```python
from build123d import *

# Parameters (mm, degrees)
SKETCH1_W           = 158.5
SKETCH1_H           = 104
SKETCH1_W_2         = 62.25
SKETCH1_H_2         = 68
BOSS_EXTRUDE1_DEPTH = 1.2
SKETCH2_W           = 4
SKETCH2_H           = 10
BOSS_EXTRUDE2_DEPTH = 2
FILLET1_R           = 2
SKETCH3_W           = 10
SKETCH3_H           = 9
BOSS_EXTRUDE3_DEPTH = 5
SKETCH4_R           = 1.3
CUT_EXTRUDE1_DEPTH  = 5
CUT_EXTRUDE2_DEPTH  = 3.8
FILLET2_R           = 5
FILLET3_R           = 2
SKETCH6_W           = 98
SKETCH6_H           = 10
BOSS_EXTRUDE4_DEPTH = 0.8
SKETCH8_W           = 16
SKETCH8_H           = 6
BOSS_EXTRUDE5_DEPTH = 2
SKETCH9_W           = 6
SKETCH9_H           = 10
SKETCH9_W_2         = 3
SKETCH9_H_2         = 9.8
BOSS_EXTRUDE6_DEPTH = 2.8
FILLET4_R           = 3
SKETCH11_W          = 10
SKETCH11_H          = 71
BOSS_EXTRUDE7_DEPTH = 2
BOSS_EXTRUDE8_DEPTH = 1.2


# Some blends are built 0.0001 mm under size
with BuildPart() as part:
    # Sketch1 → Boss-Extrude1 (new body)
    with BuildSketch(Plane(origin=(0, 0, 0), x_dir=(1, 0, 0), z_dir=(0, 1, 0))):
        with Locations((79.25, 52)):
            Rectangle(SKETCH1_W, SKETCH1_H)
        with Locations((119.375, 54)):
            Rectangle(SKETCH1_W_2, SKETCH1_H_2, mode=Mode.SUBTRACT)
        with Locations((47.125, 54)):
            Rectangle(SKETCH1_W_2, SKETCH1_H_2, mode=Mode.SUBTRACT)
    extrude(amount=BOSS_EXTRUDE1_DEPTH)

    # Sketch2 → Boss-Extrude2 (add)
    with BuildSketch(Plane.XZ):
        with Locations((149.5, -104)):
            Rectangle(SKETCH2_W, SKETCH2_H)
        with Locations((48, -104)):
            Rectangle(SKETCH2_W, SKETCH2_H)
    extrude(amount=BOSS_EXTRUDE2_DEPTH)

    # Fillet1
    fillet1_edges = [part.edges().sort_by_distance(p)[0] for p in [
        (50, 0, -101.5),
        (46, 0, -101.5),
        (147.5, 0, -101.5),
        (151.5, 0, -101.5),
    ]]
    fillet(fillet1_edges, radius=FILLET1_R - 0.0001)  # a hair under: the kernel refuses the full size

    # Sketch3 → Boss-Extrude3 (add)
    with BuildSketch(Plane(origin=(0, 0, -104), x_dir=(-1, 0, 0), z_dir=(0, 0, -1))):
        with Locations((-95.75, -3.3)):
            Rectangle(SKETCH3_W, SKETCH3_H)
    extrude(amount=-BOSS_EXTRUDE3_DEPTH)

    # Sketch4 → Cut-Extrude1 (cut)
    with BuildSketch(Plane(origin=(0, 0, -104), x_dir=(-1, 0, 0), z_dir=(0, 0, -1))):
        with Locations((-95.75, -3.3)):
            Circle(SKETCH4_R)
    extrude(amount=-CUT_EXTRUDE1_DEPTH, mode=Mode.SUBTRACT)

    # Sketch5 → Cut-Extrude2 (cut)
    with BuildSketch(Plane.XY.offset(-99)):
        with BuildLine():
            Line((92.25, -3.3), (92.25, -7.8))
            Line((92.25, -7.8), (99.25, -7.8))
            Line((99.25, -7.8), (99.25, -3.3))
            ThreePointArc((99.25, -3.3), (95.75, 0.2), (92.25, -3.3))
        make_face()
    extrude(amount=-CUT_EXTRUDE2_DEPTH, mode=Mode.SUBTRACT)

    # Fillet2
    fillet2_edges = [part.edges().sort_by_distance(p)[0] for p in [
        (100.75, 0, -101.5),
        (90.75, 0, -101.5),
    ]]
    fillet(fillet2_edges, radius=FILLET2_R)

    # Fillet3
    fillet3_edges = [part.edges().sort_by_distance(p)[0] for p in [
        (90.75, -7.8, -101.5),
        (100.75, -7.8, -101.5),
    ]]
    fillet(fillet3_edges, radius=FILLET3_R)

    # Sketch6 → Boss-Extrude4 (add)
    with BuildSketch(Plane.XZ):
        with Locations((109.5, -10.2)):
            Rectangle(SKETCH6_W, SKETCH6_H)
    extrude(amount=BOSS_EXTRUDE4_DEPTH)

    # Sketch8 → Boss-Extrude5 (add)
    with BuildSketch(Plane.XZ):
        with Locations((160.5, -10.2)):
            Rectangle(SKETCH8_W, SKETCH8_H)
    extrude(amount=BOSS_EXTRUDE5_DEPTH)

    # Sketch9 → Boss-Extrude6 (add)
    with BuildSketch(Plane.XZ):
        with Locations((155.5, -10.2)):
            Rectangle(SKETCH9_W, SKETCH9_H)
        with Locations((59, -10.1)):
            Rectangle(SKETCH9_W_2, SKETCH9_H_2)
    extrude(amount=BOSS_EXTRUDE6_DEPTH)

    # Fillet4
    # the kernel refuses this fillet: 3 mm, written as the material it adds along each edge
    with BuildSketch(Plane(origin=(57.5, 0, -5.2), x_dir=(-1, 0, 0), z_dir=(0, 0, -1))) as fillet4_piece_1:
        with BuildLine():
            CenterArc((2.993325909, -3), FILLET4_R, 90, 86.177446271)
            Line((0, -2.8), (-0.059866518, -2.796))
            ThreePointArc((-0.059866518, -2.796), (-0.06, -1.4), (-0.06, 0))
            Line((-0.06, 0), (0, 0.06))
            Line((0, 0.06), (2.993325909, 0.06))
            Line((2.993325909, 0.06), (2.993325909, 0))
        make_face()
    extrude(amount=9.8)

    # Sketch11 → Boss-Extrude7 (add)
    with BuildSketch(Plane.XZ):
        with Locations((9, -35.5)):
            Rectangle(SKETCH11_W, SKETCH11_H)
    extrude(amount=BOSS_EXTRUDE7_DEPTH)

    # Sketch12 → Boss-Extrude8 (add)
    with BuildSketch(Plane(origin=(0, 1.2, 0), x_dir=(1, 0, 0), z_dir=(0, 1, 0))):
        with BuildLine():
            Line((22.585033293, 82.977390915), (39.739539441, 64.185732728))
            ThreePointArc((39.739539441, 64.185732728), (47.125, 60.927763011), (54.510460559, 64.185732728))
            Line((54.510460559, 64.185732728), (71.664966707, 82.977390915))
            ThreePointArc((71.664966707, 82.977390915), (72.194126096, 86.210820537), (69.449328539, 88))
            Line((69.449328539, 88), (53.452699296, 88))
            Line((53.452699296, 88), (53.452699296, 91.208733434))
            Line((53.452699296, 91.208733434), (81.121703178, 91.208733434))
            Line((81.121703178, 91.208733434), (81.121703178, 63.398815268))
            Line((81.121703178, 63.398815268), (78.25, 63.398815268))
            Line((78.25, 63.398815268), (78.25, 78.263994748))
            ThreePointArc((78.25, 78.263994748), (76.334685553, 81.061039126), (73.034361832, 80.286603833))
            Line((73.034361832, 80.286603833), (55.19253522, 60.742030283))
            ThreePointArc((55.19253522, 60.742030283), (52.577995779, 54), (55.19253522, 47.257969717))
            Line((55.19253522, 47.257969717), (73.034361832, 27.713396167))
            ThreePointArc((73.034361832, 27.713396167), (76.334685553, 26.938960874), (78.25, 29.736005252))
            Line((78.25, 29.736005252), (78.25, 51.032908731))
            Line((78.25, 51.032908731), (81.121703178, 51.032908731))
            Line((81.121703178, 51.032908731), (81.121703178, 16.832253351))
            Line((81.121703178, 16.832253351), (49.123041709, 16.832253351))
            Line((49.123041709, 16.832253351), (49.123041709, 20))
            Line((49.123041709, 20), (69.449328539, 20))
            ThreePointArc((69.449328539, 20), (72.194126096, 21.789179463), (71.664966707, 25.022609085))
            Line((71.664966707, 25.022609085), (54.510460559, 43.814267272))
            ThreePointArc((54.510460559, 43.814267272), (47.125, 47.072236989), (39.739539441, 43.814267272))
            Line((39.739539441, 43.814267272), (22.585033293, 25.022609085))
            ThreePointArc((22.585033293, 25.022609085), (22.055873904, 21.789179463), (24.800671461, 20))
            Line((24.800671461, 20), (42.917495227, 20))
            Line((42.917495227, 20), (42.917495227, 16.832253351))
            Line((42.917495227, 16.832253351), (11.408469589, 16.832253351))
            Line((11.408469589, 16.832253351), (11.408469589, 46.938752597))
            Line((11.408469589, 46.938752597), (16, 46.938752597))
            Line((16, 46.938752597), (16, 29.736005252))
            ThreePointArc((16, 29.736005252), (17.915314447, 26.938960874), (21.215638168, 27.713396167))
            Line((21.215638168, 27.713396167), (39.05746478, 47.257969717))
            ThreePointArc((39.05746478, 47.257969717), (41.672004221, 54), (39.05746478, 60.742030283))
            Line((39.05746478, 60.742030283), (21.215638168, 80.286603833))
            ThreePointArc((21.215638168, 80.286603833), (17.915314447, 81.061039126), (16, 78.263994748))
            Line((16, 78.263994748), (16, 63.398815268))
            Line((16, 63.398815268), (11.408469589, 63.398815268))
            Line((11.408469589, 63.398815268), (11.408469589, 91.208733434))
            Line((11.408469589, 91.208733434), (44.179781607, 91.208733434))
            Line((44.179781607, 91.208733434), (44.179781607, 88))
            Line((44.179781607, 88), (24.800671461, 88))
            ThreePointArc((24.800671461, 88), (22.055873904, 86.210820537), (22.585033293, 82.977390915))
        make_face()
    boss_extrude8 = extrude(amount=-BOSS_EXTRUDE8_DEPTH)

    # Mirror1: Boss-Extrude8 across plane
    add(boss_extrude8.mirror(Plane(origin=(83.25, 0, 0), x_dir=(0, 0, 1), z_dir=(1, 0, 0))))


solid = part.part
```
Part model, mm, in its own coordinate system. A direction names the side the tool comes from. Coordinates: 2 decimals unless noted, no trailing zeros. Write each loop counter-clockwise with the first axis right and the second up, starting at its lowest first coordinate (ties: lowest second). Pieces come first, ordered by that corner, then holes.
Item 1: Mould opens along Z. For faces 1 (the face through (102.18, -1.5, -101.46)), 2 (the face through (47.01, 0.61, -60.93)) say: released by +Z, released by -Z, zero draft, split by the parting line, or undercut.
Item 2: Probe line 1 (Y direction, x = 95.75, z = -103.25); line 2 (Y direction, x = 8, z = -86); line 3 (X direction, y = -1.75, z = -102). List the from-to ranges inside material, lowest first.
Item 3: Slice it at B-B (z = -74.5). Write the cut outline in (x, y).
Item 4: Slice it at C-C (x = 76.5). Write the cut outline in (y, z).
Item 5: Which spindle directions (+Z, -Z, +X, -X, +Y, -Y) get a long thin tool onto all of the face, cutting with end or side? Do faces 3 (the face through (149, -2, -104)), 4 (the face through (119.26, 0.61, -47.07)), 5 (the face through (163, 0, -10)). Say none if no direction does.
Item 6: Slice it at A-A (x = 30.5). Write the cut outline in (y, z), and give its area (3 significant figures).
Item 7: Pin check, flat tips, straight feed: pin 1 (2 mm diameter, centred on x = 57, y = -2, fed in from -Z); pin 2 (2 mm diameter, centred on x = 96.5, y = -4, fed in from +Z); pin 3 (3 mm diameter, centred on x = 128, z = -11.5, fed in from -Y); pin 4 (1 mm diameter, centred on y = -2, z = -89, fed in from -X). Stop position of each tip, or through.
Results found:
1. face 1: zero draft
1. face 2: undercut
2. line 1: y = -7.8 to -4.6, -2 to 1.2
2. line 2: y = 0 to 1.2
2. line 3: x = 45.98 to 50.02, 89.55 to 92.61, 98.89 to 101.95, 147.48 to 151.52
3. outline: (0, 0) - (16, 0) - (16, 1.2) - (0, 1.2) - close; (26.5, 0) - (30.32, 0) - (30.32, 1.2) - (26.5, 1.2) - close; (63.93, 0) - (67.75, 0) - (67.75, 1.2) - (63.93, 1.2) - close; (78.25, 0) - (88.25, 0) - (88.25, 1.2) - (78.25, 1.2) - close; (98.75, 0) - (102.57, 0) - (102.57, 1.2) - (98.75, 1.2) - close; (136.18, 0) - (140, 0) - (140, 1.2) - (136.18, 1.2) - close; (150.5, 0) - (158.5, 0) - (158.5, 1.2) - (150.5, 1.2) - close
4. outline: (-0.8, -15.2) - (0, -15.2) - (0, -27.01) - (1.2, -27.01) - (1.2, 0) - (0, 0) - (0, -5.2) - (-0.8, -5.2) - close; (0, -104) - (1.2, -104) - (1.2, -80.99) - (0, -80.99) - close
5. face 3: +Z, -Z, +X, -Y
5. face 4: +Y, -Y
5. face 5: +Z, -Z, +X, +Y
6. outline: (0, -104) - (1.2, -104) - (1.2, -88) - (0, -88) - close; (0, -74.31) - (1.2, -74.31) - (1.2, -70.12) - (0, -70.12) - close; (0, -37.88) - (1.2, -37.88) - (1.2, -33.69) - (0, -33.69) - close; (0, -20) - (1.2, -20) - (1.2, 0) - (0, 0) - close
6. area: 53.3 mm2
7. pin 1: stops at z = -15
7. pin 2: stops at z = -102.8
7. pin 3: stops at y = -0.8
7. pin 4: passes through
